from build123d import *

# Parameters (mm, degrees)
F0_W     = 32
F0_H     = 32
F1_ANGLE = 57.53
F2_R     = 1.5
F3_DEPTH = 8
F4_R     = 1.5
F5_DEPTH = 8


with BuildPart() as f1:
    # F0 (on Front) → F1 (revolve)
    with BuildSketch(Plane.XZ):
        with Locations((-1.223468, 8.916048)):
            Rectangle(F0_W, F0_H)
    revolve(axis=Axis((-1.223468, 0, -7.083952), (1, 0, 0)), revolution_arc=F1_ANGLE)

    # F2 (on face) → F3 (cut)
    with BuildSketch(Plane(origin=(0, 0, 0), x_dir=(-1, 0, 0), z_dir=(0, 1, 0))):
        with Locations((-6.776532, 8.916048)):
            Circle(F2_R)
        with Locations((9.223468, 8.916048)):
            Circle(F2_R)
    extrude(amount=-F3_DEPTH, mode=Mode.SUBTRACT)

    # F4 (on face) → F5 (cut)
    with BuildSketch(Plane(origin=(0, -3.208551, -5.042241), x_dir=(1, 0, 0), z_dir=(0, -0.536858, -0.843673))):
        with Locations((6.776532, 12.196924)):
            Circle(F4_R)
        with Locations((-9.223468, 12.196924)):
            Circle(F4_R)
    extrude(amount=-F5_DEPTH, mode=Mode.SUBTRACT)


solid = f1.part
Design review of the part built by this model. Coordinates are the model's own, in mm. A direction names the side the tool comes from. Round coordinates to 2 decimals unless told otherwise and drop trailing zeros. Write each loop counter-clockwise with the first axis right and the second up, starting at its lowest first coordinate (ties: lowest second). Pieces come first, ordered by that corner, then holes. Notation, with made-up numbers: (-18, -2.5) - (23, -2.5) arc R14 ccw to (23, 20.5) - close; hole circle Ø3 at (-3.5, 14.25). An arc over 180 degrees is marked (long way). Use a Markdown table: item, result. Add a question column.
1. We need section C-C (x = 1). State the section outline as (y, z) points.
2. Mouldability with a two-part tool opening along Y and no side actions: class faces 4 (the face through (-10.329, -12.237, 5.377)), 5 (the face through (-9, -8, 9)), 6 (the face through (6.084, -3.944, 7.585)) as +Y half, -Y half, draft (parallel to the pull), parting line (faces both ways), or undercut.
3. For faces 1 (the face through (7, -8, 9)), 2 (the face through (-1.447, -13.688, 1.626)), 3 (the face through (6.756, -9.252, 8.286)), list the 3-axis set-ups (+Z, -Z, +X, -X, +Y, -Y) from which the entire face can be reached by the end or side of a thin tool; tool diameter is ignored.
4. We need section B-B (z = 15.5). State the section outline as (x, y) points, then the cut area to 3 significant figures.
5. We need section D-D (y = -18.75). State the section outline as (x, z) points, then the cut area to 3 significant figures.
6. We need section A-A (y = -5.75). State the section outline as (x, z) points, then the cut area to 3 significant figures.
7. Clearance check with flat-ended pins moving along their axes: pin 1 (10 mm diameter, centred on x = 7, y = -11.5, fed in from +Z); pin 2 (5 mm diameter, centred on x = 6, z = -3.5, fed in from -Y); pin 3 (0.9 mm diameter, centred on x = 7.5, z = 8.5, fed in from +Y). State where each tip first meets the part, or that it passes through.
8. Wall thickness on probe 1 along X at (y, z) = (-11.75, 5.5); probe 2 along Y at (x, z) = (-8, 8.5); probe 3 along Y at (x, z) = (5.5, -2): over which ranges is each line inside the solid? List them lowest first.
Output:
| question | item | result |
|---|---|---|
| 1 | outline | (-27, 10.1) - (0, -7.08) - (0, 24.92) arc R32 ccw to start |
| 2 | face 4 | undercut |
| 2 | face 5 | +Y half |
| 2 | face 6 | draft |
| 3 | face 1 | +Y |
| 3 | face 2 | -Z, +X, -X, -Y |
| 3 | face 3 | none |
| 4 | outline | (-17.22, -22.67) - (14.78, -22.67) - (14.78, 0) - (-17.22, 0) - close |
| 4 | area | 725 mm2 |
| 5 | outline | (-17.22, 4.85) - (14.78, 4.85) - (14.78, 18.85) - (-17.22, 18.85) - close |
| 5 | area | 448 mm2 |
| 6 | outline | (-17.22, -3.43) - (14.78, -3.43) - (14.78, 24.4) - (-17.22, 24.4) - close; hole circle Ø3 at (-9.22, 8.92); hole circle Ø3 at (6.78, 8.92) |
| 6 | area | 876 mm2 |
| 7 | pin 1 | stops at z = 24.25 |
| 7 | pin 2 | stops at y = -9.56 |
| 7 | pin 3 | stops at y = -8 |
| 8 | probe 1 | x = -17.22 to -10.57, -7.88 to 5.43, 8.12 to 14.78 |
| 8 | probe 2 | y = -24.49 to -10.08, -9.59 to -8 |
| 8 | probe 3 | y = -7.99 to 0 |
